from build123d import *
from build123d.topology import SkipClean

# Parameters (mm, degrees)
SKETCH1_R                     = 27.5
BOSS_EXTRUDE1_DEPTH           = 30
SKETCH4_R                     = 15
BOSS_EXTRUDE3_DEPTH           = 310
BOSS_EXTRUDE3_TAPER           = 1
BOSS_EXTRUDE3_OTHER_WAY_DEPTH = 160
SKETCH5_R                     = 12.5
BOSS_EXTRUDE4_DEPTH           = 100
FILLET1_R                     = 5
BOSS_EXTRUDE5_DEPTH           = 200
SKETCH2_R                     = 25
CUT_EXTRUDE4_DEPTH            = 20
CUT_EXTRUDE6_DEPTH            = 50


with BuildPart() as part:
    # Sketch1 → Boss-Extrude1 (new body)
    with BuildSketch(Plane(origin=(0, 0, 0), x_dir=(1, 0, 0), z_dir=(0, 1, 0))):
        with Locations(Location((0, 0, 0), (0, 0, 270))):
            Circle(SKETCH1_R)
    extrude(amount=BOSS_EXTRUDE1_DEPTH)

    # Sketch4 → Boss-Extrude3 (add)
    with BuildSketch(Plane(origin=(0, 0, 0), x_dir=(0, 0, -1), z_dir=(1, 0, 0))):
        with Locations((0, 15)):
            Circle(SKETCH4_R)
    extrude(amount=BOSS_EXTRUDE3_DEPTH, taper=BOSS_EXTRUDE3_TAPER)

    # Sketch4 → Boss-Extrude3 other way (add)
    with SkipClean():  # the faces are left unmerged after this step: merging them gives an invalid solid
        with BuildSketch(Plane(origin=(0, 0, 0), x_dir=(0, 0, -1), z_dir=(1, 0, 0))):
            with Locations((0, 15)):
                Circle(SKETCH4_R)
        extrude(amount=-BOSS_EXTRUDE3_OTHER_WAY_DEPTH)

    # Sketch5 → Boss-Extrude4 (add)
    with SkipClean():  # the faces are left unmerged after this step: merging them gives an invalid solid
        with BuildSketch(Plane.ZY.offset(160)):
            with Locations((0, 15)):
                Circle(SKETCH5_R)
        extrude(amount=BOSS_EXTRUDE4_DEPTH)

    # Fillet1
    fillet1_edges = [part.edges().sort_by_distance(p)[0] for p in [
        (-260, 15, -12.5),
    ]]
    fillet(fillet1_edges, radius=FILLET1_R)

    # Sketch7 → Boss-Extrude5 (add)
    with SkipClean():  # the faces are left unmerged after this step: merging them gives an invalid solid
        with BuildSketch(Plane(origin=(0, 15, 0), x_dir=(1, 0, 0), z_dir=(0, 1, 0))):
            Polygon((26, -14.546168312), (26, 14.546168312), (310, 0), align=None)
        extrude(amount=BOSS_EXTRUDE5_DEPTH)

    # Sketch2 → Cut-Extrude4 (cut)
    with SkipClean():  # the faces are left unmerged after this step: merging them gives an invalid solid
        with BuildSketch(Plane.XZ):
            with Locations(Location((0, 0, 0), (0, 0, 270))):
                Circle(SKETCH2_R)
        extrude(amount=-CUT_EXTRUDE4_DEPTH, mode=Mode.SUBTRACT)

    # Sketch9 → Cut-Extrude6 (cut)
    with SkipClean():  # the faces are left unmerged after this step: merging them gives an invalid solid
        with BuildSketch(Plane(origin=(0.811118683, 0, -15.836315168), x_dir=(-0.9986908871720133, 0, -0.0511518511842649), z_dir=(0.0511518511842649, 0, -0.9986908871720134))):
            Polygon((-25.22189963, 29.762241759), (-125.22189963, 215), (-25.22189963, 215), align=None)
        extrude(amount=-CUT_EXTRUDE6_DEPTH, mode=Mode.SUBTRACT)


solid = part.part
Can you work these out from the model? Positions are in its coordinate system, mm. A direction names the side the tool comes from. Round coordinates to 2 decimals unless told otherwise and drop trailing zeros. Loops run counter-clockwise (first coordinate to the right, second up) from the corner with the lowest first, then second, coordinate; pieces in that order, holes last. Notation, with made-up numbers: (17, 85.25) - (44, 85.25) arc R32 ccw to (44, 120.25) - close; hole circle Ø6 at (-5, -12). An arc over 180 degrees is marked (long way). Write item = value, one per line. Start each with the question number.
(1) If I drill on probe 1 along Z at (x, y) = (0, 6); probe 2 along X at (y, z) = (13, 0); probe 3 along X at (y, z) = (6, 0), over which ranges is the centre line in solid material (lowest first)? Write a range as [from, to].
(2) If we section it at C-C (y = 160): Please give me the cut outline in (x, z), and give its area (3 significant figures).
(3) If we section it at A-A (x = -73): Please give me the cut outline in (y, z).
(4) If we section it at B-B (x = -204): Please give me the cut outline in (y, z).
(5) For faces 1 (the face through (-206.84, 3.91, 5.77)), 2 (the face through (7.509, 9.86, -23.846)), 3 (the face through (197.57, 113.6, -5.76)), 4 (the face through (169.99, 113.6, 7.17)), which set-ups out of +Z, -Z, +X, -X, +Y, -Y let a thin tool reach every point of the face, with its end or its side?
(6) If we mould it in two halves opening along X, with no side actions, what happens to faces 5 (the face through (0, 20, 0)), 6 (the face through (-1, 30, 0)), 7 (the face through (26, 30.2, 2.2)), 8 (the face through (-160, 27.3, 3.4))? For each: released by +X, released by -X, zero draft, split by the parting line, or undercut.
(7) For P1, Ø12, axis at x = -2.5, z = -9.5, coming from the -Y side; P2, Ø12, axis at x = -135.5, z = 18, coming from the -Y side; P3, Ø2, axis at x = -152, z = 9, coming from the +Y side, each with a flat end and sliding along its axis, tell me the tip position at first contact or that it passes through.
(8) If we section it at D-D (y = 62): Please give me the cut outline in (x, z), and give its area (3 significant figures).
Ans:
q1.probe_1 = [-27.5, -25], [25, 27.5]
q1.probe_2 = [-260, -25], [25, 310]
q1.probe_3 = [-259.77, -25], [25, 310]
q2.outline = (95.09, 11.01) - (96.22, -10.95) - (310, 0) - close
q2.area = 2,350 mm²
q3.outline = circle Ø30 at (15, 0)
q4.outline = circle Ø25 at (15, 0)
q5.face_1 = -X
q5.face_2 = -Y
q5.face_3 = -Z, +X, +Y
q5.face_4 = +Z, +X, +Y
q6.face_5 = undercut
q6.face_6 = zero draft
q6.face_7 = undercut
q6.face_8 = released by -X
q7.P1 = 20
q7.P2 = 6
q7.P3 = 27.69
q8.outline = (41.98, 13.73) - (43.38, -13.66) - (310, 0) - close
q8.area = 3,660 mm²
